Input: part model. Units: mm. Frame: model coordinates. Face numbers are marked on the shaded views. A direction names the side the tool comes from. Give positions to 0.01 mm unless a question says otherwise; leave off trailing zeros. Use a Markdown table: item, result.
from build123d import *

# Parameters (mm, degrees)
SKETCH1_W                      = 45
SKETCH1_H                      = 26.6
BOSS_EXTRUDE1_DEPTH            = 3
SKETCH3_W                      = 15.5
SKETCH3_H                      = 3
CUT_EXTRUDE1_DEPTH             = 2
SKETCH4_W                      = 15.5
SKETCH4_H                      = 1.5
CUT_EXTRUDE2_DEPTH             = 53.312140082
FILLET1_SIZE                   = 3
BOSS_EXTRUDE2_REACH            = 54.36
SKETCH5_R                      = 0.75
SKETCH6_W                      = 18.5
SKETCH6_H                      = 10.6
CUT_EXTRUDE3_DEPTH             = 53.359908383
CUT_EXTRUDE4_DEPTH             = 2
CUT_EXTRUDE5_REACH             = 52.901
SKETCH8_W                      = 5.25
SKETCH8_H                      = 0.5
CUT_EXTRUDE5_DIRECTION_2_REACH = 52.901
CUT_EXTRUDE6_REACH             = 52.901
SKETCH9_W                      = 5.25
SKETCH9_H                      = 0.5
CUT_EXTRUDE6_DIRECTION_2_REACH = 52.901
FILLET2_R                      = 0.8
FILLET3_R                      = 5
SKETCH10_W                     = 11.5
SKETCH10_H                     = 20.6
CUT_EXTRUDE7_DEPTH             = 53.359908383
FILLET4_R                      = 5
FILLET5_R                      = 0.5


with BuildPart() as part:
    # Sketch1 → Boss-Extrude1 (new body)
    with BuildSketch(Plane(origin=(0, 0, 0), x_dir=(1, 0, 0), z_dir=(0, 1, 0))):
        with Locations((22.5, 13.3)):
            Rectangle(SKETCH1_W, SKETCH1_H)
    extrude(amount=BOSS_EXTRUDE1_DEPTH)

    # Sketch3 → Cut-Extrude1 (cut)
    with BuildSketch(Plane(origin=(0, 3, 0), x_dir=(1, 0, 0), z_dir=(0, 1, 0))):
        with Locations((15.75, 25.1)):
            Rectangle(SKETCH3_W, SKETCH3_H)
        with Locations((15.75, 1.5)):
            Rectangle(SKETCH3_W, SKETCH3_H)
    extrude(amount=-CUT_EXTRUDE1_DEPTH, mode=Mode.SUBTRACT)

    # Sketch4 → Cut-Extrude2 (cut, through all)
    with BuildSketch(Plane(origin=(0, 1, 0), x_dir=(1, 0, 0), z_dir=(0, 1, 0))):
        with Locations((15.75, 0.75)):
            Rectangle(SKETCH4_W, SKETCH4_H)
        with Locations((15.75, 25.85)):
            Rectangle(SKETCH4_W, SKETCH4_H)
    extrude(amount=-CUT_EXTRUDE2_DEPTH, mode=Mode.SUBTRACT)

    # Fillet1
    # a fillet whose section is not a circle: 3 mm, written as the material it takes off along each edge
    with BuildSketch(Plane(origin=(0, 3, -34.1), x_dir=(1, 0, 0), z_dir=(0, 0, 1))) as fillet1_piece_1:
        with BuildLine():
            Bezier((FILLET1_SIZE, 0), (0, 0), (0, -FILLET1_SIZE), weights=[1, 0.212132034, 1])
            Line((0, -FILLET1_SIZE), (0, 0))
            Line((0, 0), (FILLET1_SIZE, 0))
        make_face()
    extrude(amount=41.6, mode=Mode.SUBTRACT)

    # Sketch5 → Boss-Extrude2 (add, up to next)
    with BuildSketch(Plane(origin=(0, 3, 0), x_dir=(1, 0, 0), z_dir=(0, 1, 0)), mode=Mode.PRIVATE) as boss_extrude2_sk1:
        with Locations((19, 3)):
            Circle(SKETCH5_R)
    boss_extrude2_tool1 = extrude(boss_extrude2_sk1.sketch, amount=-BOSS_EXTRUDE2_REACH, mode=Mode.PRIVATE) - part.part
    # Sketch5 → Boss-Extrude2 (add, up to next)
    with BuildSketch(Plane(origin=(0, 3, 0), x_dir=(1, 0, 0), z_dir=(0, 1, 0)), mode=Mode.PRIVATE) as boss_extrude2_sk2:
        with Locations((19, 23.6)):
            Circle(SKETCH5_R)
    boss_extrude2_tool2 = extrude(boss_extrude2_sk2.sketch, amount=-BOSS_EXTRUDE2_REACH, mode=Mode.PRIVATE) - part.part
    add(boss_extrude2_tool1.solids().sort_by_distance((19, 3, -3))[0])
    add(boss_extrude2_tool2.solids().sort_by_distance((19, 3, -23.6))[0])

    # Sketch6 → Cut-Extrude3 (cut, through all)
    with BuildSketch(Plane(origin=(0, 3, 0), x_dir=(1, 0, 0), z_dir=(0, 1, 0))):
        with Locations((17.25, 13.3)):
            Rectangle(SKETCH6_W, SKETCH6_H)
    extrude(amount=-CUT_EXTRUDE3_DEPTH, mode=Mode.SUBTRACT)

    # Sketch7 → Cut-Extrude4 (cut)
    with BuildSketch(Plane(origin=(0, 3, 0), x_dir=(1, 0, 0), z_dir=(0, 1, 0))):
        Polygon((18.25, 3), (16.5, 3), (16.5, 6), (23.5, 6), (23.5, 4.25), (18.25, 4.25), align=None)
        Polygon((18.25, 22.35), (18.25, 23.6), (16.5, 23.6), (16.5, 20.6), (23.5, 20.6), (23.5, 22.35), align=None)
    extrude(amount=-CUT_EXTRUDE4_DEPTH, mode=Mode.SUBTRACT)

    # Sketch8 → Cut-Extrude5 (cut, up to next)
    with BuildSketch(Plane.XY.offset(-3), mode=Mode.PRIVATE) as cut_extrude5_sk1:
        with Locations((20.875, 1.25)):
            Rectangle(SKETCH8_W, SKETCH8_H)
    cut_extrude5_tool1 = extrude(cut_extrude5_sk1.sketch, amount=-CUT_EXTRUDE5_REACH, mode=Mode.PRIVATE) & part.part
    add(cut_extrude5_tool1.solids().sort_by_distance((20.875, 1.25, -3))[0], mode=Mode.SUBTRACT)

    # Sketch8 → Cut-Extrude5 direction 2 (cut, up to next)
    with BuildSketch(Plane.XY.offset(-3), mode=Mode.PRIVATE) as cut_extrude5_direction_2_sk1:
        with Locations((20.875, 1.25)):
            Rectangle(SKETCH8_W, SKETCH8_H)
    cut_extrude5_direction_2_tool1 = extrude(cut_extrude5_direction_2_sk1.sketch, amount=CUT_EXTRUDE5_DIRECTION_2_REACH, mode=Mode.PRIVATE) & part.part
    add(cut_extrude5_direction_2_tool1.solids().sort_by_distance((20.875, 1.25, -3))[0], mode=Mode.SUBTRACT)

    # Sketch9 → Cut-Extrude6 (cut, up to next)
    with BuildSketch(Plane(origin=(0, 0, -23.6), x_dir=(-1, 0, 0), z_dir=(0, 0, -1)), mode=Mode.PRIVATE) as cut_extrude6_sk1:
        with Locations((-20.875, 1.25)):
            Rectangle(SKETCH9_W, SKETCH9_H)
    cut_extrude6_tool1 = extrude(cut_extrude6_sk1.sketch, amount=-CUT_EXTRUDE6_REACH, mode=Mode.PRIVATE) & part.part
    add(cut_extrude6_tool1.solids().sort_by_distance((20.875, 1.25, -23.6))[0], mode=Mode.SUBTRACT)

    # Sketch9 → Cut-Extrude6 direction 2 (cut, up to next)
    with BuildSketch(Plane(origin=(0, 0, -23.6), x_dir=(-1, 0, 0), z_dir=(0, 0, -1)), mode=Mode.PRIVATE) as cut_extrude6_direction_2_sk1:
        with Locations((-20.875, 1.25)):
            Rectangle(SKETCH9_W, SKETCH9_H)
    cut_extrude6_direction_2_tool1 = extrude(cut_extrude6_direction_2_sk1.sketch, amount=CUT_EXTRUDE6_DIRECTION_2_REACH, mode=Mode.PRIVATE) & part.part
    add(cut_extrude6_direction_2_tool1.solids().sort_by_distance((20.875, 1.25, -23.6))[0], mode=Mode.SUBTRACT)

    # Fillet2
    fillet2_edges = [part.edges().sort_by_distance(p)[0] for p in [
        (18.25, 2.25, -4.25),
        (18.25, 2.25, -22.35),
    ]]
    fillet(fillet2_edges, radius=FILLET2_R)

    # Fillet3
    fillet3_edges = [part.edges().sort_by_distance(p)[0] for p in [
        (45, 1.5, -26.6),
        (45, 1.5, 0),
    ]]
    fillet(fillet3_edges, radius=FILLET3_R)

    # Sketch10 → Cut-Extrude7 (cut, through all)
    with BuildSketch(Plane(origin=(0, 3, 0), x_dir=(1, 0, 0), z_dir=(0, 1, 0))):
        with Locations((36.25, 13.3)):
            Rectangle(SKETCH10_W, SKETCH10_H)
    extrude(amount=-CUT_EXTRUDE7_DEPTH, mode=Mode.SUBTRACT)

    # Fillet4
    fillet4_edges = [part.edges().sort_by_distance(p)[0] for p in [
        (42, 1.5, -23.6),
        (42, 1.5, -3),
        (30.5, 1.5, -3),
        (30.5, 1.5, -23.6),
    ]]
    fillet(fillet4_edges, radius=FILLET4_R)

    # Fillet5
    fillet5_edges = [part.edges().sort_by_distance(p)[0] for p in [
        (23.5, 2, -6),
        (16.5, 2, -6),
        (16.5, 2, -3),
        (16.5, 2, -23.6),
        (16.5, 2, -20.6),
        (23.5, 2, -20.6),
        (23.5, 2.25, -4.25),
        (23.5, 2.25, -22.35),
    ]]
    fillet(fillet5_edges, radius=FILLET5_R)


solid = part.part
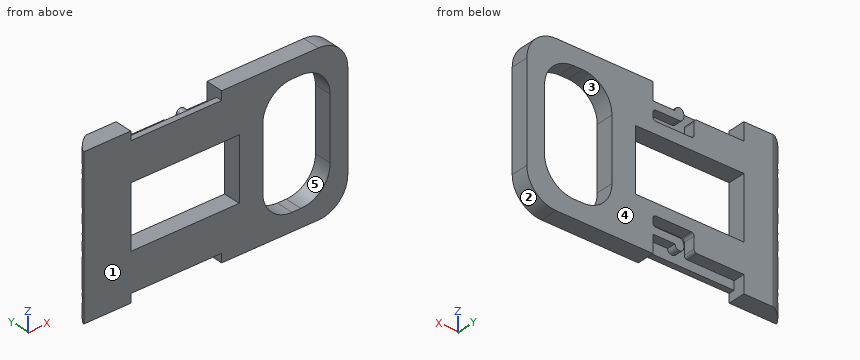
1) Material intervals for line 1 (Z direction, x = 21.5, y = 2.45); line 2 (Z direction, x = 36, y = 2.9); line 3 (Z direction, x = 10.5, y = 0.85), sorted ascending. Write a range as from..to.
Response values:
| item | result |
|---|---|
| line 1 | z = -23.6..-22.35, -20.6..-18.6, -8..-6, -4.25..-3 |
| line 2 | z = -26.6..-23.6, -3..0 |
| line 3 | z = -25.1..-18.6, -8..-1.5 |
2) First-contact query: pin 1 Ø1.6 at (x, y) = (11, 2) entering from +Z; pin 2 Ø0.6 at (x, y) = (10, 2.5) entering from -Z; pin 3 Ø0.9 at (y, z) = (1, -13.5) entering from -X. Flat tips, straight axial feed; report the tip coordinate or a pass-through.
Response values:
| item | result |
|---|---|
| pin 1 | stops at z = -3 |
| pin 2 | stops at z = -23.6 |
| pin 3 | stops at x = 0.23 |
3) Cut plane A-A on z = -9.25. State how many separate pieces and enclosed holes the cut face has, and give its area (3 significant figures).
Response values:
| item | result |
|---|---|
| separate pieces | 3 |
| enclosed holes | 0 |
| area | 41.7 mm² |
4) Mould query, pull axis Z, two halves, no side actions, for the marked faces 1, 2 and 3. Classes: released by +Z, released by -Z, zero draft, split by the parting line, or undercut.
Response values:
| item | result |
|---|---|
| face 1 | zero draft |
| face 2 | released by -Z |
| face 3 | undercut |
5) Reachability of the marked faces 4 and 5 from +Z, -Z, +X, -X, +Y, -Y: full face, straight path, thin tool, end or side. Return the list, or none.
Response values:
| item | result |
|---|---|
| face 4 | +Z, -Z, +X, -X, +Y |
| face 5 | +Y, -Y |
